```python
from build123d import *

# Parameters (mm, degrees)
SKETCH_1_R          = 0.65
SKETCH_1_R_2        = 1.5
EXTRUDE_1_DEPTH     = 2.3
SKETCH_2_R          = 4.4
EXTRUDE_2_DEPTH     = 3.2
SKETCH_3_R          = 4.4
SKETCH_3_R_2        = 3.4
SKETCH_3_R_3        = 2.75
SKETCH_3_R_4        = 1.5
CUT_EXTRUDE_1_DEPTH = 1


with BuildPart() as part:
    # Эскиз1 → Бобышка-Вытянуть1 (new body)
    with BuildSketch(Plane.XY):
        with BuildLine():
            Line((-3.968626967, 4.5), (-16.888114198, 2.469689731))
            ThreePointArc((-16.888114198, 2.469689731), (-19, 0), (-16.888114198, -2.469689731))
            Line((-16.888114198, -2.469689731), (-3.968626967, -4.5))
            ThreePointArc((-3.968626967, -4.5), (0, -6), (3.968626967, -4.5))
            Line((3.968626967, -4.5), (16.888114198, -2.469689731))
            ThreePointArc((16.888114198, -2.469689731), (19, 0), (16.888114198, 2.469689731))
            Line((16.888114198, 2.469689731), (3.968626967, 4.5))
            ThreePointArc((3.968626967, 4.5), (0, 6), (-3.968626967, 4.5))
        make_face()
        with Locations((-16.5, 0)):
            Circle(SKETCH_1_R, mode=Mode.SUBTRACT)
        with Locations((-13.5, 0)):
            Circle(SKETCH_1_R, mode=Mode.SUBTRACT)
        with Locations((-10.5, 0)):
            Circle(SKETCH_1_R, mode=Mode.SUBTRACT)
        with Locations((-7.5, 0)):
            Circle(SKETCH_1_R, mode=Mode.SUBTRACT)
        with Locations((16.5, 0)):
            Circle(SKETCH_1_R, mode=Mode.SUBTRACT)
        with Locations((7.5, 0)):
            Circle(SKETCH_1_R, mode=Mode.SUBTRACT)
        with Locations((10.5, 0)):
            Circle(SKETCH_1_R, mode=Mode.SUBTRACT)
        with Locations((13.5, 0)):
            Circle(SKETCH_1_R, mode=Mode.SUBTRACT)
        Circle(SKETCH_1_R_2, mode=Mode.SUBTRACT)
    extrude(amount=EXTRUDE_1_DEPTH)

    # Эскиз2 → Бобышка-Вытянуть2 (add)
    with BuildSketch(Plane.XY.offset(2.3)):
        Circle(SKETCH_2_R)
        Polygon((0.333439775, 2.639447604), (0, 3.05), (-0.333439775, 2.639447604), (-0.758504156, 2.954178641), (-0.979368078, 2.473601404), (-1.469348706, 2.672735374), (-1.563759083, 2.15232973), (-2.087868673, 2.223354314), (-2.049893354, 1.695819264), (-2.575200173, 1.634271725), (-2.407225286, 1.132754236), (-2.900722375, 0.942501833), (-2.6133024, 0.498514094), (-3.043981522, 0.191511085), (-2.655176114, -0.167049522), (-2.995976115, -0.571513009), (-2.530215347, -0.822116802), (-2.75972251, -1.298626839), (-2.246271844, -1.42552746), (-2.35006539, -1.944143169), (-1.821186821, -1.939366985), (-1.792745019, -2.467501833), (-1.281669931, -2.33134895), (-1.122779886, -2.835818282), (-0.661621006, -2.576843686), (-0.382266362, -3.025949839), (0, -2.660425857), (0.382266362, -3.025949839), (0.661621006, -2.576843686), (1.122779886, -2.835818282), (1.281669931, -2.33134895), (1.792745019, -2.467501833), (1.821186821, -1.939366985), (2.35006539, -1.944143169), (2.246271844, -1.42552746), (2.75972251, -1.298626839), (2.530215347, -0.822116802), (2.995976115, -0.571513009), (2.655176114, -0.167049522), (3.043981522, 0.191511085), (2.6133024, 0.498514094), (2.900722375, 0.942501833), (2.407225286, 1.132754236), (2.575200173, 1.634271725), (2.049893354, 1.695819264), (2.087868673, 2.223354314), (1.563759083, 2.15232973), (1.469348706, 2.672735374), (0.979368078, 2.473601404), (0.758504156, 2.954178641), align=None, mode=Mode.SUBTRACT)
    extrude(amount=EXTRUDE_2_DEPTH)

    # Эскиз3 → Вырез-Вытянуть1 (cut)
    with BuildSketch(Plane(origin=(0, 0, 0), x_dir=(-1, 0, 0), z_dir=(0, 0, -1))):
        Circle(SKETCH_3_R)
        Circle(SKETCH_3_R_2, mode=Mode.SUBTRACT)
        Circle(SKETCH_3_R_3)
        Circle(SKETCH_3_R_4, mode=Mode.SUBTRACT)
    extrude(amount=-CUT_EXTRUDE_1_DEPTH, mode=Mode.SUBTRACT)


solid = part.part
```
Geometry check sheet. Reference: the model listing, model coordinates, mm. A direction names the side the tool comes from. Give positions to 0.01 mm unless a question says otherwise; leave off trailing zeros. Order: outer loops, then holes, each group sorted by start corner. A loop starts at its lowest first (then second) coordinate and runs counter-clockwise, first axis right, second up.
1. Section check C-C, the plane x = 10.5. Enter the section's corners in (y, z).
2. Thickness scan on L1, parallel to Y at x = 0, z = 0.45; L2, parallel to Y at x = 0, z = 2.05; L3, parallel to Y at x = -16.5, z = 1.1. Record the ranges inside material, lowest first.
3. Release check for a two-part mould opening along X. For faces 1 (the face through (-19, 0, 1)), 2 (the face through (10.52, 3.47, 1.13)), 3 (the face through (-2, -3, 1)) record: pulls with the +X half, pulls with the -X half, needs draft (parallel to the pull), parting line crosses it, or undercut.
4. Section check A-A, the plane z = 1.85. Give the number of separate pieces and of enclosed holes in the cut face, and give its area (3 significant figures).
5. Access from +Z, -Z, +X, -X, +Y, -Y to the whole of each face (thin tool, end or side, straight path). Record for faces 4 (the face through (-4.197, 1.322, 0.493)), 5 (the face through (6.85, 0.03, 1.13)), 6 (the face through (-1.4, 1.4, 2.3)).
6. Section check B-B, the plane x = 16.5. Enter the section's corners in (y, z).
7. Section check D-D, the plane y = -5. Enter the section's corners in (x, z), and give its area (3 significant figures).
8. Gauge pin test, flat ends, axial feed: pin 1 Ø2 at (x, y) = (7, -3.5) entering from +Z; pin 2 Ø1.6 at (x, y) = (1.5, 1) entering from -Z; pin 3 Ø3 at (x, z) = (9, 3.5) entering from +Y. Record the tip position at first contact, or that the pin passes through.
Values follow:
1. outline: (-3.47, 0) - (-0.65, 0) - (-0.65, 2.3) - (-3.47, 2.3) - close; (0.65, 0) - (3.47, 0) - (3.47, 2.3) - (0.65, 2.3) - close
2. L1: y = -6 to -4.4, -3.4 to -2.75, 2.75 to 3.4, 4.4 to 6
2. L2: y = -6 to -1.5, 1.5 to 6
2. L3: y = -2.53 to -0.65, 0.65 to 2.53
3. face 1: pulls with the -X half
3. face 2: pulls with the +X half
3. face 3: undercut
4. separate pieces: 1
4. enclosed holes: 9
4. area: 266 mm2
5. face 4: -Z
5. face 5: +Z, -Z
5. face 6: +Z
6. outline: (-2.53, 0) - (-0.65, 0) - (-0.65, 2.3) - (-2.53, 2.3) - close; (0.65, 0) - (2.53, 0) - (2.53, 2.3) - (0.65, 2.3) - close
7. outline: (-3.32, 0) - (3.32, 0) - (3.32, 2.3) - (-3.32, 2.3) - close
7. area: 15.3 mm2
8. pin 1: stops at z = 2.3
8. pin 2: stops at z = 1
8. pin 3: stops at y = 3.85
